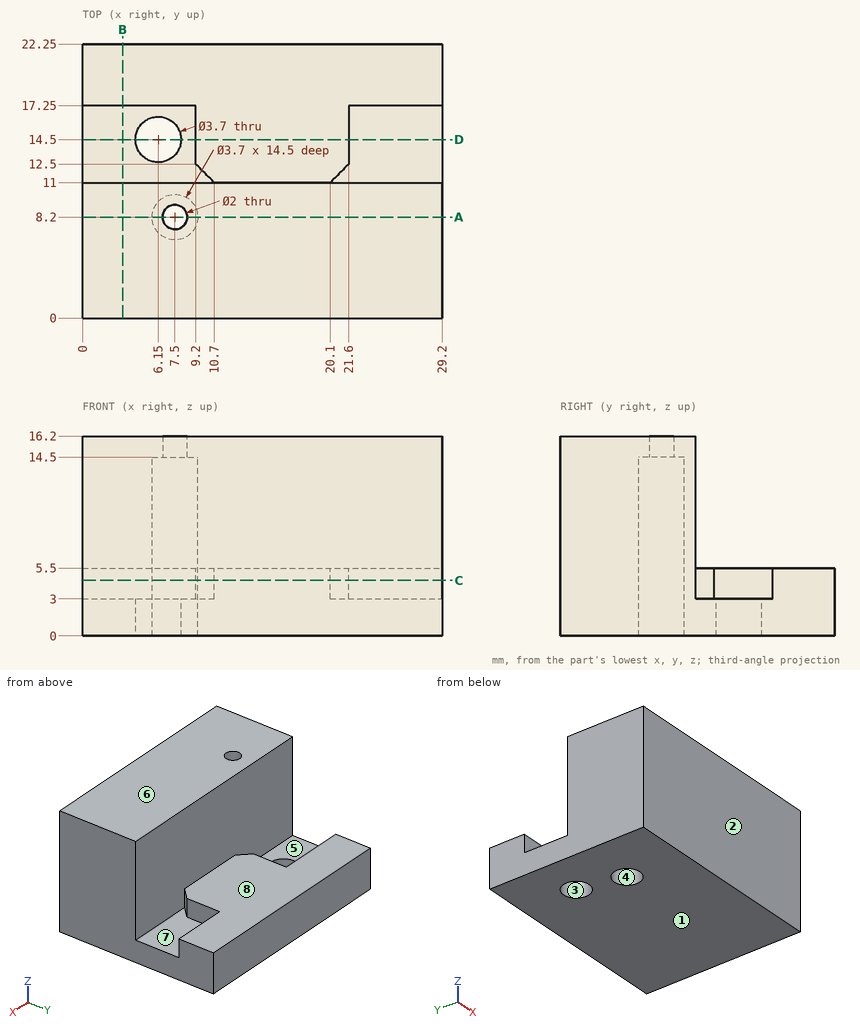
Study the drawing (mm; zero at the part's minimum x, y, z) and answer. A direction names the side the tool comes from. Give positions to 0.01 mm unless a question says otherwise; leave off trailing zeros. Loops run counter-clockwise (first coordinate to the right, second up) from the corner with the lowest first, then second, coordinate; pieces in that order, holes last. Notation, with made-up numbers: (3.25, 60) - (43.25, 60) arc R24 ccw to (43.25, 96) - close; hole circle Ø2 at (52, -10.75). An arc over 180 degrees is marked (long way). Use CSV: the item, a comma, the result in double quotes. Start each with the question number.
(1) Find section D-D, the plane y = 14.5. Determine the outline of the cut face in (x, z).
(2) A tool of negligible diameter and unlimited length cuts with its end or side. For the marked faces 4, 5, 6, 7 and 8, from which of +Z, -Z, +X, -X, +Y, -Y can it reach the whole face along a straight path? Write none if from no direction.
(3) Each of these flat-tipped pins is pushed along its axis until it touches: pin 1 (5 mm diameter, centred on x = 6.15, y = 14.5, fed in from +Z); pin 2 (6 mm diameter, centred on x = 26, z = 10, fed in from +Y); pin 3 (7 mm diameter, centred on x = 24.5, y = 15, fed in from +Z). Where does it stop, or does it pass through?
(4) Determine the mould class of the marked faces 1, 2 and 3 for opening direction Y: released by +Y, released by -Y, zero draft, split by the parting line, or undercut.
(5) Find the intervals of material crossed by L1, parallel to Y at x = 7.5, z = 3.5; L2, parallel to Y at x = 7.5, z = 6.75; L3, parallel to Z at x = 17.5, y = 17.5, in increasing order.
(6) Find section B-B, the plane x = 3.25. Determine the outline of the cut face in (y, z), plus the area to 3 significant figures.
(7) Find section C-C, the plane z = 4.5. Determine the outline of the cut face in (x, y), plus the area to 3 significant figures.
(8) Find section A-A, the plane y = 8.2. Determine the outline of the cut face in (x, z).
Results found:
1,outline,"(0, 0) - (4.3, 0) - (4.3, 3) - (0, 3) - close; (8, 0) - (29.2, 0) - (29.2, 3) - (21.6, 3) - (21.6, 5.5) - (9.2, 5.5) - (9.2, 3) - (8, 3) - close"
2,face 4,"-Z"
2,face 5,"+Z, -X"
2,face 6,"+Z, +X, -X, +Y, -Y"
2,face 7,"+Z, +X"
2,face 8,"+Z, +X, -X, +Y"
3,pin 1,"z = 3"
3,pin 2,"y = 11"
3,pin 3,"z = 5.5"
4,face 1,"zero draft"
4,face 2,"released by -Y"
4,face 3,"undercut"
5,L1,"0 to 6.35, 10.05 to 11, 17.25 to 22.25"
5,L2,"0 to 6.35, 10.05 to 11"
5,L3,"0 to 5.5"
6,outline,"(0, 0) - (22.25, 0) - (22.25, 5.5) - (17.25, 5.5) - (17.25, 3) - (11, 3) - (11, 16.2) - (0, 16.2) - close"
6,area,"224 mm^2"
7,outline,"(0, 0) - (29.2, 0) - (29.2, 11) - (20.1, 11) - (21.6, 12.5) - (21.6, 17.25) - (29.2, 17.25) - (29.2, 22.25) - (0, 22.25) - (0, 17.25) - (9.2, 17.25) - (9.2, 12.5) - (10.7, 11) - (0, 11) - close; hole circle Ø3.7 at (7.5, 8.2)"
7,area,"532 mm^2"
8,outline,"(0, 0) - (5.65, 0) - (5.65, 14.5) - (6.5, 14.5) - (6.5, 16.2) - (0, 16.2) - close; (8.5, 14.5) - (9.35, 14.5) - (9.35, 0) - (29.2, 0) - (29.2, 16.2) - (8.5, 16.2) - close"
